Can you work these out from the model? Positions are in its coordinate system, mm. A direction names the side the tool comes from. Round coordinates to 2 decimals unless told otherwise and drop trailing zeros. Loops run counter-clockwise (first coordinate to the right, second up) from the corner with the lowest first, then second, coordinate; pieces in that order, holes last.
from build123d import *

# Parameters (mm, degrees)
F3_DEPTH = 25.4


with BuildPart() as f1:
    # F0 (on Front) → F1 (revolve)
    with BuildSketch(Plane.XZ):
        Polygon((31.75, 12.7), (0, 12.7), (0, 0), (50.8, 0), (50.8, 7.9375), (31.75, 7.9375), align=None)
    revolve(axis=Axis((24.74322, 0, 0), (1, 0, 0)))

    # F2 (on face) → F3 (cut)
    with BuildSketch(Plane(origin=(0, 0, 0), x_dir=(0, -1, 0), z_dir=(-1, 0, 0))):
        with BuildLine():
            ThreePointArc((7.62, 10.16), (0, 12.7), (-7.62, 10.16))
            Line((-7.62, 10.16), (7.62, 10.16))
        make_face()
        with BuildLine():
            Line((7.62, -10.16), (-7.62, -10.16))
            ThreePointArc((-7.62, -10.16), (0, -12.7), (7.62, -10.16))
        make_face()
    extrude(amount=-F3_DEPTH, mode=Mode.SUBTRACT)


solid = f1.part
(1) For faces 1 (the flat face through (31.75, 8.3, 0.2)), 2 (the flat face through (13, 0, -10.16)), 3 (the flat face through (50.8, 0, 0)), 4 (the flat face through (25.4, 0, 11)), which set-ups out of +Z, -Z, +X, -X, +Y, -Y let a thin tool reach every point of the face, with its end or its side?
Worked answers:
face 1: +X
face 2: -Z, -X, +Y, -Y
face 3: +Z, -Z, +X, +Y, -Y
face 4: +Z, -X, +Y, -Y
(2) Will these pins go through, and if not, where does the flat tip stop? P1, Ø0.8, axis at y = 0.5, z = 12, coming from the -X side; P2, Ø6, axis at x = 25.5, y = 2.5, coming from the +Z side; P3, Ø4, axis at x = 8, y = -6, coming from the +Z side; P4, Ø12, axis at x = 38.5, y = 1, coming from the +Z side.
Worked answers:
P1: stops at x = 25.4
P2: stops at z = 12.7
P3: stops at z = 10.16
P4: stops at z = 7.94
(3) If I drill on line 1 (Z direction, x = 6, y = 0); line 2 (Z direction, x = 48, y = 0); line 3 (Y direction, x = 3.5, z = -0.5), over which ranges is the centre line in solid material (lowest first)?
Worked answers:
line 1: z = -10.16 to 10.16
line 2: z = -7.94 to 7.94
line 3: y = -12.69 to 12.69
(4) If we section it at D-D, the plane y = 3.75: List the corners of the cut face in (x, z) for me, then the cut area to 3 significant figures.
Worked answers:
outline: (0, -10.16) - (25.4, -10.16) - (25.4, -12.13) - (31.75, -12.13) - (31.75, -7) - (50.8, -7) - (50.8, 7) - (31.75, 7) - (31.75, 12.13) - (25.4, 12.13) - (25.4, 10.16) - (0, 10.16) - close
area: 937 mm2
(5) If we section it at A-A, the plane z = 0: List the corners of the cut face in (x, y) for me, then the cut area to 3 significant figures.
Worked answers:
outline: (0, -12.7) - (31.75, -12.7) - (31.75, -7.94) - (50.8, -7.94) - (50.8, 7.94) - (31.75, 7.94) - (31.75, 12.7) - (0, 12.7) - close
area: 1,110 mm2
(6) If we section it at B-B, the plane y = 0: List the corners of the cut face in (x, z) for me, then the cut area to 3 significant figures.
Worked answers:
outline: (0, -10.16) - (25.4, -10.16) - (25.4, -12.7) - (31.75, -12.7) - (31.75, -7.94) - (50.8, -7.94) - (50.8, 7.94) - (31.75, 7.94) - (31.75, 12.7) - (25.4, 12.7) - (25.4, 10.16) - (0, 10.16) - close
area: 980 mm2
(7) If we section it at C-C, the plane x = 6.5: List the corners of the cut face in (y, z) for me.
Worked answers:
outline: (-7.62, -10.16) - (7.62, -10.16) arc R12.7 ccw to (7.62, 10.16) - (-7.62, 10.16) arc R12.7 ccw to start
